```python
from build123d import *

# Parameters (mm, degrees)
F1_DEPTH = 5
F2_W     = 47
F2_H     = 27
F3_DEPTH = 25
F4_W     = 15
F4_H     = 5
F5_DEPTH = 15
F6_R     = 3
F7_DEPTH = 25
F6_R_2   = 5
F8_DEPTH = 1.5


with BuildPart() as f1:
    # F0 (on Top) → F1 (new body)
    with BuildSketch(Plane.XY):
        with BuildLine():
            Line((-35, -22.5), (35, -22.5))
            Line((35, -22.5), (35, 12.5))
            ThreePointArc((35, 12.5), (32.071068, 19.571068), (25, 22.5))
            Line((25, 22.5), (-25, 22.5))
            ThreePointArc((-25, 22.5), (-32.071068, 19.571068), (-35, 12.5))
            Line((-35, 12.5), (-35, -22.5))
        make_face()
    extrude(amount=F1_DEPTH)

    # F2 (on Top) → F3 (cut)
    with BuildSketch(Plane.XY):
        Rectangle(F2_W, F2_H)
    extrude(amount=F3_DEPTH, mode=Mode.SUBTRACT)

    # F4 (on face) → F5 (join)
    with BuildSketch(Plane.XY.offset(5)):
        with Locations((-27.5, -20)):
            Rectangle(F4_W, F4_H)
        with Locations((27.5, -20)):
            Rectangle(F4_W, F4_H)
    extrude(amount=F5_DEPTH)

    # F6 (on face) → F7 (cut)
    with BuildSketch(Plane(origin=(0, -17.5, 0), x_dir=(-1, 0, 0), z_dir=(0, 1, 0))):
        with Locations((27.5, 12.5)):
            Circle(F6_R)
        with Locations((-27.5, 12.5)):
            Circle(F6_R)
    extrude(amount=-F7_DEPTH, mode=Mode.SUBTRACT)

    # F6 (on face) → F8 (cut)
    with BuildSketch(Plane(origin=(0, -17.5, 0), x_dir=(-1, 0, 0), z_dir=(0, 1, 0))):
        with Locations((27.5, 12.5)):
            Circle(F6_R_2)
        with Locations((27.5, 12.5)):
            Circle(F6_R, mode=Mode.SUBTRACT)
        with Locations((-27.5, 12.5)):
            Circle(F6_R_2)
        with Locations((-27.5, 12.5)):
            Circle(F6_R, mode=Mode.SUBTRACT)
    extrude(amount=-F8_DEPTH, mode=Mode.SUBTRACT)


solid = f1.part
```
Input: part model. Units: mm. Frame: model coordinates. A direction names the side the tool comes from. Give positions to 0.01 mm unless a question says otherwise; leave off trailing zeros. Write each loop counter-clockwise with the first axis right and the second up, starting at its lowest first coordinate (ties: lowest second). Pieces come first, ordered by that corner, then holes. Notation, with made-up numbers: (19.5, 59.25) - (26.5, 59.25) arc R19 cw to (26.5, 89.25) - close; hole circle Ø9 at (-16, -39.5). An arc over 180 degrees is marked (long way). Write item = value, one per line. Start each with the question number.
1. Section query B-B, the plane z = 12.5. Output: boundary loops of the cut face in (x, y), then the cut area to 3 significant figures.
2. First-contact query: pin 1 Ø4 at (x, z) = (13, 5.5) entering from +Y; pin 2 Ø4.5 at (x, z) = (-30, 13.5) entering from +Y; pin 3 Ø6 at (x, y) = (-16.5, 9) entering from +Z; pin 4 Ø8 at (x, z) = (-25.5, 13.5) entering from +Y. Flat tips, straight axial feed; report the tip coordinate or a pass-through.
3. Section query D-D, the plane x = 27.5. Output: boundary loops of the cut face in (y, z), then the cut area to 3 significant figures.
4. Mould query, pull axis Z, two halves, no side actions, for faces 1 (the flat face through (25, -19, 10)), 2 (the flat face through (-23.5, 0, 2)), 3 (the flat face through (0, -15, 0)). Classes: released by +Z, released by -Z, zero draft, split by the parting line, or undercut.
5. Access query for faces 4 (the flat face through (-20, -20, 12)), 5 (the flat face through (-30, -19, 10)), 6 (the flat face through (0, 13.5, 2)), 7 (the flat face through (-28, -17.5, 7)). Directions: +Z, -Z, +X, -X, +Y, -Y. A direction counts if a zero-diameter tool reaches every point of the face in a straight line with its end or side. Return the directions, or none.
6. Ray query, L1, parallel to Z at x = 27.5, y = -18.05; L2, parallel to Z at x = -27.5, y = -20.9; L3, parallel to Y at x = 26.5, z = 6.75. Return the intervals inside material, ascending.
7. Section query C-C, the plane z = 2.25. Output: boundary loops of the cut face in (x, y).
8. Section query A-A, the plane y = 7.5. Output: boundary loops of the cut face in (x, z), then the cut area to 3 significant figures.
Check sheet entries:
q1.outline = (-35, -22.5) - (-30.5, -22.5) - (-30.5, -19) - (-32.5, -19) - (-32.5, -17.5) - (-35, -17.5) - close; (-24.5, -22.5) - (-20, -22.5) - (-20, -17.5) - (-22.5, -17.5) - (-22.5, -19) - (-24.5, -19) - close; (20, -22.5) - (24.5, -22.5) - (24.5, -19) - (22.5, -19) - (22.5, -17.5) - (20, -17.5) - close; (30.5, -22.5) - (35, -22.5) - (35, -17.5) - (32.5, -17.5) - (32.5, -19) - (30.5, -19) - close
q1.area = 78.0 mm2
q2.pin_1 = 22.5
q2.pin_2 = -19
q2.pin_3 = through
q2.pin_4 = -17.5
q3.outline = (-22.5, 0) - (22.18, 0) - (22.18, 5) - (-17.5, 5) - (-17.5, 7.5) - (-19, 7.5) - (-19, 9.5) - (-22.5, 9.5) - close; (-22.5, 15.5) - (-19, 15.5) - (-19, 17.5) - (-17.5, 17.5) - (-17.5, 20) - (-22.5, 20) - close
q3.area = 262 mm2
q4.face_1 = undercut
q4.face_2 = zero draft
q4.face_3 = released by -Z
q5.face_4 = +Z, +Y, -Y
q5.face_5 = +Y
q5.face_6 = +Z, -Z
q5.face_7 = +Z, +X, -X, +Y
q6.L1 = 0 to 7.5, 17.5 to 20
q6.L2 = 0 to 9.5, 15.5 to 20
q6.L3 = -22.5 to -17.5
q7.outline = (-35, -22.5) - (35, -22.5) - (35, 12.5) arc R10 ccw to (25, 22.5) - (-25, 22.5) arc R10 ccw to (-35, 12.5) - close; hole (-23.5, -13.5) - (23.5, -13.5) - (23.5, 13.5) - (-23.5, 13.5) - close
q8.outline = (-35, 0) - (-23.5, 0) - (-23.5, 5) - (-35, 5) - close; (23.5, 0) - (35, 0) - (35, 5) - (23.5, 5) - close
q8.area = 115 mm2
